from build123d import *

# Parameters (mm, degrees)
SKETCH033_R     = 1.75
SKETCH033_R_2   = 4.796418
SKETCH033_R_3   = 6.720156
PAD001_DEPTH    = 3
CHAMFER001_SIZE = 2
CHAMFER002_SIZE = 1.4


with BuildPart() as part:
    # Sketch033 → Pad001 (new body)
    with BuildSketch(Plane(origin=(0, -38, 0), x_dir=(1, 0, 0), z_dir=(0, -0.939693, 0.34202))):
        with BuildLine():
            Line((-34.406356, 37.6), (34.406361, 37.6))
            ThreePointArc((42.400003, 29.918894), (39.949322, 35.368499), (34.406361, 37.6))
            Line((42.400003, 29.918894), (43.15, 11.118894))
            ThreePointArc((35.156359, 2.8), (40.924857, 5.257038), (43.15, 11.118894))
            Line((35.156359, 2.8), (-35.156359, 2.8))
            ThreePointArc((-43.15, 11.118896), (-40.924858, 5.257039), (-35.156359, 2.8))
            Line((-43.15, 11.118896), (-42.399997, 29.918896))
            ThreePointArc((-34.406356, 37.6), (-39.949317, 35.368499), (-42.399997, 29.918896))
        make_face()
        with Locations((-36.75, 32.3)):
            Circle(SKETCH033_R, mode=Mode.SUBTRACT)
        with Locations((36.75, 32.3)):
            Circle(SKETCH033_R, mode=Mode.SUBTRACT)
        with Locations((-38, 8.3)):
            Circle(SKETCH033_R, mode=Mode.SUBTRACT)
        with Locations((38, 8.3)):
            Circle(SKETCH033_R, mode=Mode.SUBTRACT)
        with Locations((-29.768274, 20.799871)):
            Circle(SKETCH033_R_2, mode=Mode.SUBTRACT)
        with Locations((27.980227, 19.489883)):
            Circle(SKETCH033_R_3, mode=Mode.SUBTRACT)
        with BuildLine():
            Line((-13.009558, 27.89562), (13.133726, 27.89562))
            ThreePointArc((16.384062, 24.645284), (15.43206, 26.943619), (13.133726, 27.89562))
            Line((16.384062, 24.645284), (16.384062, 12.013562))
            ThreePointArc((13.393686, 9.023187), (15.508201, 9.899048), (16.384062, 12.013562))
            Line((13.393686, 9.023187), (-13.746031, 9.023187))
            ThreePointArc((-17.177177, 12.454333), (-16.172218, 10.028147), (-13.746031, 9.023187))
            Line((-17.177177, 12.454333), (-17.177177, 23.728001))
            ThreePointArc((-13.009558, 27.89562), (-15.95651, 26.674953), (-17.177177, 23.728001))
        make_face(mode=Mode.SUBTRACT)
    extrude(amount=PAD001_DEPTH)

    # Chamfer001
    chamfer001_edges = [part.edges().sort_by_distance(p)[0] for p in [
        (0.062084, -31.278214, 27.239369),
    ]]
    chamfer(chamfer001_edges, length=CHAMFER001_SIZE)

    # Chamfer002
    chamfer002_edges = [part.edges().sort_by_distance(p)[0] for p in [
        (-38.5, -29.771827, 31.378132),
        (-39.75, -37.980311, 8.825509),
        (35, -29.771827, 31.378132),
        (36.25, -37.980311, 8.825509),
    ]]
    chamfer(chamfer002_edges, length=CHAMFER002_SIZE)


solid = part.part
Build history of the part. All positions in model axes, mm. A direction names the side the tool comes from. Give positions to 0.01 mm unless a question says otherwise; leave off trailing zeros. Loops run counter-clockwise (first coordinate to the right, second up) from the corner with the lowest first, then second, coordinate; pieces in that order, holes last. Notation, with made-up numbers: (-13.5, 58.25) - (35.5, 58.25) arc R15 cw to (35.5, 75.25) - close; hole circle Ø11 at (-31.5, -7). An arc over 180 degrees is marked (long way). Write item = value, one per line. Start each with the question number.
1) Band-saw the part on D-D on x = -31. Give the cut face in (y, z).
2) Pull direction X, two halves, no side cores. Call faces 5 (the flat face through (-0.48, -26.53, 35.84)), 6 (the cylindrical face through (34.19, -33.6, 16.4)), 7 (the cylindrical face through (-40.99, -37.57, 5.51)): +X half, -X half, draft (parallel to the pull), parting line (faces both ways), or undercut.
3) Probe probe 1 along Y at (x, z) = (-23.5, 4); probe 2 along X at (y, z) = (-34.25, 15); probe 3 along Y at (x, z) = (2.5, 30). List the from-to ranges inside material, lowest first. Write a range as from..to.
4) Band-saw the part on C-C on x = -21.5. Give the cut face in (y, z), plus the area to 3 significant figures.
5) Tool access for faces 1 (the conical face through (-16.7, -36.46, 9.48)), 2 (the conical face through (15.96, -30.266, 26.487)), 3 (the cylindrical face through (15.485, -35.086, 9.449)), 4 (the cylindrical face through (15.46, -29.26, 25.46)): list every direction of +Z, -Z, +X, -X, +Y, -Y with a clear straight run to the whole face (end or side of a thin tool).
6) Drop flat-ended pins along their axis: pin 1 Ø2 at (x, z) = (18.5, 8.5) entering from +Y; pin 2 Ø5 at (x, z) = (-6.5, 28) entering from +Y; pin 3 Ø4 at (x, z) = (16, 23.5) entering from -Y. Give the stop position or say it passes through.
7) Band-saw the part on B-B on z = 17.5. Count the separate pieces of the cut face and the enclosed holes in it, plus the area to 3 significant figures.
8) Band-saw the part on A-A on x = -7.5. Give the cut face in (y, z), plus the area to 3 significant figures.
Final values:
q1.outline = (-39.86, 3.66) - (-37.04, 2.63) - (-32.47, 15.19) - (-35.29, 16.22) - close; (-32.12, 24.93) - (-29.3, 23.9) - (-25.14, 35.33) - (-27.96, 36.36) - close
q2.face_5 = draft
q2.face_6 = undercut
q2.face_7 = -X half
q3.probe_1 = -39.74..-36.54
q3.probe_2 = -42.98..-17.78, 16.99..22.66, 33.3..42.98
q3.probe_3 = -30.27..-27.08
q4.outline = (-39.86, 3.66) - (-37.04, 2.63) - (-25.14, 35.33) - (-27.96, 36.36) - close
q4.area = 104 mm²
q5.face_1 = +Z, -Y
q5.face_2 = -Y
q5.face_3 = +Z, +Y
q5.face_4 = -Z, -Y
q6.pin_1 = -34.54
q6.pin_2 = -26.9
q6.pin_3 = -32.35
q7.separate_pieces = 4
q7.enclosed_holes = 0
q7.area = 95.3 mm²
q8.outline = (-39.86, 3.66) - (-37.04, 2.63) - (-34.91, 8.48) - (-35.85, 8.82) - (-38.42, 7.63) - close; (-30.59, 29.12) - (-29.4, 26.56) - (-28.46, 26.21) - (-25.14, 35.33) - (-27.96, 36.36) - close
q8.area = 43.8 mm²
